Check sheet for the modelled part. Datum: model origin and axes. Units: mm. A direction names the side the tool comes from. Round coordinates to 2 decimals unless told otherwise and drop trailing zeros. Write each loop counter-clockwise with the first axis right and the second up, starting at its lowest first coordinate (ties: lowest second). Pieces come first, ordered by that corner, then holes.
Item 1: Release check for a two-part mould opening along Y. For faces 6 (the flat face through (-1, 50, 2)), 7 (the flat face through (15, 8, -11)), 8 (the cylindrical face through (-0.78, -9.05, 2.54)) record: +Y half, -Y half, draft (parallel to the pull), parting line (faces both ways), or undercut.
Item 2: Material ranges on line 1 (Z direction, x = -37, y = 8.5); line 2 (X direction, y = -0.5, z = -13); line 3 (Y direction, x = 0, z = 3.35), recorded low to high.
Item 3: Tool access check on faces 1 (the flat face through (3, -18, 0)), 2 (the cylindrical face through (0.423, -11.778, -15.21)), 3 (the flat face through (-15, 9, -11)), 4 (the flat face through (50, -1, 2)), 5 (the cylindrical face through (0, -30, -15)). Record the directions out of +Z, -Z, +X, -X, +Y, -Y that give a thin tool (end or side, any length) a straight path to the whole face; none if there is none.
Item 4: Cross-section at A-A on x = 0. Enter the section's corners in (y, z).
Item 5: Go/stop test with flat-tipped pins: pin 1 Ø8 at (y, z) = (39.5, -7) entering from -X; pin 2 Ø2 at (x, z) = (-15, -6) entering from +Y; pin 3 Ø15 at (y, z) = (26, -14) entering from +X. Record where each tip stops, or that it passes through.
Item 6: Cross-section at C-C on y = 39. Enter the section's corners in (x, z), plus the area to 3 significant figures.
Item 7: Cross-section at B-B on z = -23.5. Enter the section's corners in (x, y), plus the area to 3 significant figures.
Item 8: Cross-section at D-D on x = 18. Enter the section's corners in (y, z), plus the area to 3 significant figures.
from build123d import *

# Parameters (mm, degrees)
ESQUISSE1_W             = 100
ESQUISSE1_H             = 100
BOSS_EXTRU_1_DEPTH      = 5
BOSS_EXTRU_2_DEPTH      = 30
ENL_V_MAT_EXTRU_1_DEPTH = 30
ESQUISSE6_R             = 3.25
ENL_V_MAT_EXTRU_2_DEPTH = 35
ESQUISSE7_R             = 6
ENL_V_MAT_EXTRU_3_DEPTH = 5


with BuildPart() as part:
    # Esquisse1 → Boss.-Extru.1 (new body)
    with BuildSketch(Plane.XY):
        Rectangle(ESQUISSE1_W, ESQUISSE1_H)
    extrude(amount=BOSS_EXTRU_1_DEPTH)

    # Esquisse4 → Boss.-Extru.2 (add)
    with BuildSketch(Plane(origin=(0, 0, 0), x_dir=(-1, 0, 0), z_dir=(0, 0, -1))):
        with BuildLine():
            Line((-15, 45), (15, 45))
            Line((15, 45), (15, -15))
            ThreePointArc((15, -15), (0, -30), (-15, -15))
            Line((-15, -15), (-15, 45))
        make_face()
    extrude(amount=BOSS_EXTRU_2_DEPTH)

    # Esquisse5 → Enlèv. mat.-Extru.1 (cut)
    with BuildSketch(Plane(origin=(15, 0, 0), x_dir=(0, 0, -1), z_dir=(1, 0, 0))):
        Polygon((0, 45), (30, 0), (30, 45), align=None)
    extrude(amount=-ENL_V_MAT_EXTRU_1_DEPTH, mode=Mode.SUBTRACT)

    # Esquisse6 → Enlèv. mat.-Extru.2 (cut)
    with BuildSketch(Plane(origin=(0, 0, -30), x_dir=(-1, 0, 0), z_dir=(0, 0, -1))):
        with Locations((0, -15)):
            Circle(ESQUISSE6_R)
    extrude(amount=-ENL_V_MAT_EXTRU_2_DEPTH, mode=Mode.SUBTRACT)

    # Esquisse7 → Enlèv. mat.-Extru.3 (cut)
    with BuildSketch(Plane.XY.offset(5)):
        with Locations((0, -15)):
            Circle(ESQUISSE7_R)
    extrude(amount=-ENL_V_MAT_EXTRU_3_DEPTH, mode=Mode.SUBTRACT)


solid = part.part
Response values:
1. face 6: +Y half
1. face 7: draft
1. face 8: undercut
2. line 1: z = 0 to 5
2. line 2: x = -15 to 15
2. line 3: y = -50 to -21, -9 to 50
3. face 1: +Z
3. face 2: +Z, -Z
3. face 3: -Z, -X, +Y, -Y
3. face 4: +Z, -Z, +X, +Y, -Y
3. face 5: -Z, -Y
4. outline: (-50, 0) - (-30, 0) - (-30, -30) - (-18.25, -30) - (-18.25, 0) - (-21, 0) - (-21, 5) - (-50, 5) - close; (-11.75, -30) - (0, -30) - (45, 0) - (50, 0) - (50, 5) - (-9, 5) - (-9, 0) - (-11.75, 0) - close
5. pin 1: stops at x = -15
5. pin 2: stops at y = 37.5
5. pin 3: stops at x = 15
6. outline: (-50, 0) - (-15, 0) - (-15, -4) - (15, -4) - (15, 0) - (50, 0) - (50, 5) - (-50, 5) - close
6. area: 620 mm2
7. outline: (-15, -15) arc R15 ccw to (15, -15) - (15, 9.75) - (-15, 9.75) - close; hole circle Ø6.5 at (0, -15)
7. area: 1,060 mm2
8. outline: (-50, 0) - (50, 0) - (50, 5) - (-50, 5) - close
8. area: 500 mm2
